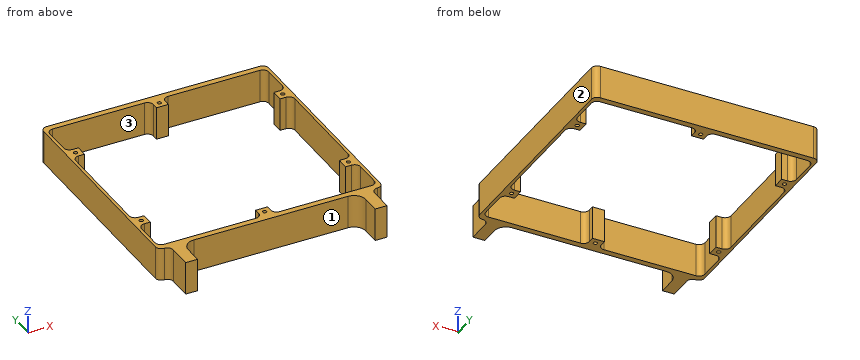
```python
from build123d import *

# Parameters (mm, degrees)
F0_R     = 1.016
F1_DEPTH = 17.78


with BuildPart() as f1:
    # F0 (on Top) → F1 (new body)
    with BuildSketch(Plane.XY):
        with BuildLine():
            Line((57.15, 60.325), (-57.15, 60.325))
            ThreePointArc((-57.15, 60.325), (-59.395064, 59.395064), (-60.325, 57.15))
            Line((-60.325, 57.15), (-60.325, -57.15))
            ThreePointArc((-60.325, -57.15), (-59.395064, -59.395064), (-57.15, -60.325))
            ThreePointArc((-57.15, -60.325), (-54.904936, -61.254936), (-53.975, -63.5))
            Line((-53.975, -63.5), (-53.975, -76.2))
            Line((-53.975, -76.2), (-47.625, -76.2))
            Line((-47.625, -76.2), (-47.625, -66.675))
            ThreePointArc((-47.625, -66.675), (-45.765128, -62.184872), (-41.275, -60.325))
            Line((-41.275, -60.325), (41.275, -60.325))
            ThreePointArc((41.275, -60.325), (45.765128, -62.184872), (47.625, -66.675))
            Line((47.625, -66.675), (47.625, -76.2))
            Line((47.625, -76.2), (53.975, -76.2))
            Line((53.975, -76.2), (53.975, -63.5))
            ThreePointArc((53.975, -63.5), (54.904936, -61.254936), (57.15, -60.325))
            ThreePointArc((57.15, -60.325), (59.395064, -59.395064), (60.325, -57.15))
            Line((60.325, -57.15), (60.325, 57.15))
            ThreePointArc((60.325, 57.15), (59.395064, 59.395064), (57.15, 60.325))
        make_face()
        with Locations((-55.5625, -33.655)):
            Circle(F0_R, mode=Mode.SUBTRACT)
        with Locations((0, -53.975)):
            Circle(F0_R, mode=Mode.SUBTRACT)
        with Locations((55.5625, -33.655)):
            Circle(F0_R, mode=Mode.SUBTRACT)
        with Locations((-55.5625, 33.655)):
            Circle(F0_R, mode=Mode.SUBTRACT)
        with BuildLine():
            ThreePointArc((-58.7375, 53.975), (-57.807564, 56.220064), (-55.5625, 57.15))
            Line((-55.5625, 57.15), (-6.35, 57.15))
            ThreePointArc((-6.35, 57.15), (-4.104936, 56.220064), (-3.175, 53.975))
            Line((-3.175, 53.975), (-3.175, 50.8))
            Line((-3.175, 50.8), (3.175, 50.8))
            Line((3.175, 50.8), (3.175, 53.975))
            ThreePointArc((3.175, 53.975), (4.104936, 56.220064), (6.35, 57.15))
            Line((6.35, 57.15), (55.5625, 57.15))
            ThreePointArc((55.5625, 57.15), (57.807564, 56.220064), (58.7375, 53.975))
            Line((58.7375, 53.975), (58.7375, 40.005))
            ThreePointArc((58.7375, 40.005), (57.807564, 37.759936), (55.5625, 36.83))
            Line((55.5625, 36.83), (52.3875, 36.83))
            Line((52.3875, 36.83), (52.3875, 30.48))
            Line((52.3875, 30.48), (55.5625, 30.48))
            ThreePointArc((55.5625, 30.48), (57.807564, 29.550064), (58.7375, 27.305))
            Line((58.7375, 27.305), (58.7375, -27.305))
            ThreePointArc((58.7375, -27.305), (57.807564, -29.550064), (55.5625, -30.48))
            Line((55.5625, -30.48), (52.3875, -30.48))
            Line((52.3875, -30.48), (52.3875, -36.83))
            Line((52.3875, -36.83), (55.5625, -36.83))
            ThreePointArc((55.5625, -36.83), (57.807564, -37.759936), (58.7375, -40.005))
            Line((58.7375, -40.005), (58.7375, -53.975))
            ThreePointArc((58.7375, -53.975), (57.807564, -56.220064), (55.5625, -57.15))
            Line((55.5625, -57.15), (6.35, -57.15))
            ThreePointArc((6.35, -57.15), (4.104936, -56.220064), (3.175, -53.975))
            Line((3.175, -53.975), (3.175, -50.8))
            Line((3.175, -50.8), (-3.175, -50.8))
            Line((-3.175, -50.8), (-3.175, -53.975))
            ThreePointArc((-3.175, -53.975), (-4.104936, -56.220064), (-6.35, -57.15))
            Line((-6.35, -57.15), (-55.5625, -57.15))
            ThreePointArc((-55.5625, -57.15), (-57.807564, -56.220064), (-58.7375, -53.975))
            Line((-58.7375, -53.975), (-58.7375, -40.005))
            ThreePointArc((-58.7375, -40.005), (-57.807564, -37.759936), (-55.5625, -36.83))
            Line((-55.5625, -36.83), (-52.3875, -36.83))
            Line((-52.3875, -36.83), (-52.3875, -30.48))
            Line((-52.3875, -30.48), (-55.5625, -30.48))
            ThreePointArc((-55.5625, -30.48), (-57.807564, -29.550064), (-58.7375, -27.305))
            Line((-58.7375, -27.305), (-58.7375, 27.305))
            ThreePointArc((-58.7375, 27.305), (-57.807564, 29.550064), (-55.5625, 30.48))
            Line((-55.5625, 30.48), (-52.3875, 30.48))
            Line((-52.3875, 30.48), (-52.3875, 36.83))
            Line((-52.3875, 36.83), (-55.5625, 36.83))
            ThreePointArc((-55.5625, 36.83), (-57.807564, 37.759936), (-58.7375, 40.005))
            Line((-58.7375, 40.005), (-58.7375, 53.975))
        make_face(mode=Mode.SUBTRACT)
        with Locations((0, 53.975)):
            Circle(F0_R, mode=Mode.SUBTRACT)
        with Locations((55.5625, 33.655)):
            Circle(F0_R, mode=Mode.SUBTRACT)
    extrude(amount=F1_DEPTH)


solid = f1.part
```
Geometry check sheet. Reference: the model listing, model coordinates, mm. Face numbers are marked on the shaded views. A direction names the side the tool comes from. Coordinates: 2 decimals unless noted, no trailing zeros. Order: outer loops, then holes, each group sorted by start corner. A loop starts at its lowest first (then second) coordinate and runs counter-clockwise, first axis right, second up.
Item 1: Scan lines: line 1 along Y through (x, z) = (0, 7) (3 decimals); line 2 along X through (y, z) = (-69, 7.5) (3 decimals); line 3 along X through (y, z) = (1.5, 7.25) (1 decimal). Record each from-to range of solid material in increasing order.
Item 2: Section check A-A (y = 5). Enter the section's corners in (x, z) (1 decimal), plus the area to 3 significant figures.
Item 3: Section check B-B (x = 24). Enter the section's corners in (y, z) (3 decimals), plus the area to 3 significant figures.
Item 4: Depth check by flat-ended pin: pin 1 (8 mm diameter, centred on x = -5, z = 2, fed in from -Y) (3 decimals); pin 2 (10.5 mm diameter, centred on y = -69, z = 8.5, fed in from +X) (3 decimals). Enter the tip coordinate at first touch or a pass-through.
Item 5: Section check C-C (z = 14.25). Count the separate pieces of the cut face and the enclosed holes in it, plus the area to 3 significant figures.
Item 6: Tool access check on the marked faces 1, 2 and 3. Record the directions out of +Z, -Z, +X, -X, +Y, -Y that give a thin tool (end or side, any length) a straight path to the whole face; none if there is none.
Check sheet entries:
1. line 1: y = -60.325 to -54.991, -52.959 to -50.8, 50.8 to 52.959, 54.991 to 60.325
1. line 2: x = -53.975 to -47.625, 47.625 to 53.975
1. line 3: x = -60.3 to -58.7, 58.7 to 60.3
2. outline: (-60.3, 0) - (-58.7, 0) - (-58.7, 17.8) - (-60.3, 17.8) - close; (58.7, 0) - (60.3, 0) - (60.3, 17.8) - (58.7, 17.8) - close
2. area: 56.5 mm2
3. outline: (-60.325, 0) - (-57.15, 0) - (-57.15, 17.78) - (-60.325, 17.78) - close; (57.15, 0) - (60.325, 0) - (60.325, 17.78) - (57.15, 17.78) - close
3. area: 113 mm2
4. pin 1: stops at y = -60.325
4. pin 2: stops at x = 53.975
5. separate pieces: 1
5. enclosed holes: 7
5. area: 1,600 mm2
6. face 1: +Z, -Z, -Y
6. face 2: +Z, -Z, +X, +Y, -Y
6. face 3: +Z, -Z
